```python
from build123d import *

# Parameters (mm, degrees)
SKETCH1_W           = 19.81
SKETCH1_H           = 6.73
BOSS_EXTRUDE1_DEPTH = 7.37
SKETCH2_W           = 1.57
SKETCH2_H           = 0.25
BOSS_EXTRUDE2_DEPTH = 2.79
CHAMFER1_SIZE       = 0.4
SKETCH3_W           = 17.31
SKETCH3_H           = 4.23
CUT_EXTRUDE1_DEPTH  = 6
FILLET1_R           = 0.5


with BuildPart() as part:
    # Sketch1 → Boss-Extrude1 (new body)
    with BuildSketch(Plane(origin=(0, 0, 0), x_dir=(1, 0, 0), z_dir=(0, 1, 0))):
        with Locations((9.905, 3.365)):
            Rectangle(SKETCH1_W, SKETCH1_H)
    extrude(amount=BOSS_EXTRUDE1_DEPTH)

    # Sketch2 → Boss-Extrude2 (add)
    with BuildSketch(Plane.XZ):
        with Locations((3.17, -5.065)):
            Rectangle(SKETCH2_W, SKETCH2_H)
        with Locations((3.17, -1.665)):
            Rectangle(SKETCH2_W, SKETCH2_H)
        with Locations((16.64, -1.665)):
            Rectangle(SKETCH2_W, SKETCH2_H)
        with Locations((16.64, -5.065)):
            Rectangle(SKETCH2_W, SKETCH2_H)
    extrude(amount=BOSS_EXTRUDE2_DEPTH)

    # Chamfer1
    chamfer1_edges = [part.edges().sort_by_distance(p)[0] for p in [
        (3.955, -2.79, -5.065),
        (2.385, -2.79, -5.065),
        (3.955, -2.79, -1.665),
        (2.385, -2.79, -1.665),
        (17.425, -2.79, -1.665),
        (15.855, -2.79, -1.665),
        (17.425, -2.79, -5.065),
        (15.855, -2.79, -5.065),
    ]]
    chamfer(chamfer1_edges, length=CHAMFER1_SIZE)

    # Sketch3 → Cut-Extrude1 (cut)
    with BuildSketch(Plane(origin=(0, 7.37, 0), x_dir=(1, 0, 0), z_dir=(0, 1, 0))):
        with Locations((9.905, 3.365)):
            Rectangle(SKETCH3_W, SKETCH3_H)
    extrude(amount=-CUT_EXTRUDE1_DEPTH, mode=Mode.SUBTRACT)

    # Fillet1
    fillet1_edges = [part.edges().sort_by_distance(p)[0] for p in [
        (19.81, 7.37, -3.365),
        (9.905, 7.37, -6.73),
        (0, 7.37, -3.365),
        (0, 3.685, -6.73),
        (19.81, 3.685, -6.73),
        (19.81, 3.685, 0),
        (0, 3.685, 0),
        (9.905, 7.37, 0),
    ]]
    fillet(fillet1_edges, radius=FILLET1_R)


solid = part.part
```
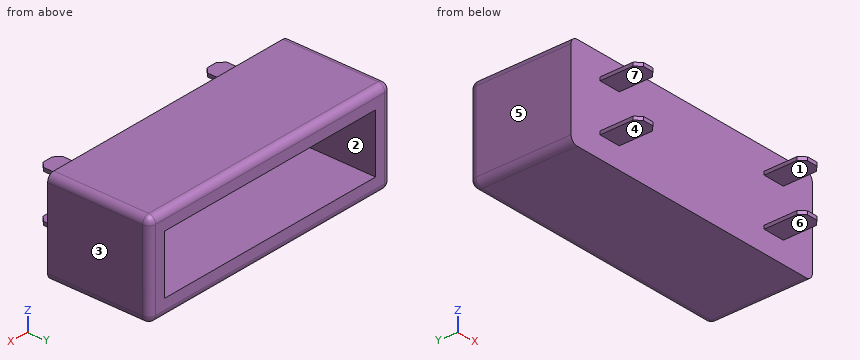
CAD build for the part. Positions are in the model's coordinates, mm. Face numbers are marked on the shaded views. A direction names the side the tool comes from. Round coordinates to 2 decimals unless told otherwise and drop trailing zeros. Order: outer loops, then holes, each group sorted by start corner. A loop starts at its lowest first (then second) coordinate and runs counter-clockwise, first axis right, second up. Notation, with made-up numbers: (-31, -26) - (11, -26) arc R13 cw to (11, -3) - close; hole circle Ø9 at (5, -5.5). An arc over 180 degrees is marked (long way). Answer as CSV lines item,"result". Start each with the question number.
1. Pin check, flat tips, straight feed: pin 1 (0.5 mm diameter, centred on x = 3.5, y = -1.5, fed in from -Z); pin 2 (1.5 mm diameter, centred on y = -1, z = -3, fed in from +X); pin 3 (1.3 mm diameter, centred on x = 16.5, y = -1.5, fed in from +Z). Stop position of each tip, or through.
2. Saw through at A-A, the plane y = 2.75. Write the cut outline in (x, z), and give its area (3 significant figures).
3. Saw through at B-B, the plane x = 6.5. Write the cut outline in (y, z), and give its area (3 significant figures).
4. Tool access for the marked faces 1, 2, 3 and 4: list every direction of +Z, -Z, +X, -X, +Y, -Y with a clear straight run to the whole face (end or side of a thin tool).
5. Drill centre lines: L1, parallel to X at y = 5, z = -4.25; L2, parallel to Z at x = 17, y = 4.75; L3, parallel to Y at x = 9.5, z = -4. Where is each one in solid material? Low to high. Write a range as [from, to].
6. Pull direction Z, two halves, no side cores. Call the marked faces 5, 6 and 7: +Z half, -Z half, draft (parallel to the pull), parting line (faces both ways), or undercut.
7. Saw through at C-C, the plane y = -0.25. Write the cut outline in (x, z) (3 decimals).
8. Saw through at D-D, the plane z = -4.25. Write the cut outline in (x, y).
Model answer:
1,pin 1,"stops at z = -5.19"
1,pin 2,"passes through"
1,pin 3,"stops at z = -1.54"
2,outline,"(0, -6.23) arc R0.5 ccw to (0.5, -6.73) - (19.31, -6.73) arc R0.5 ccw to (19.81, -6.23) - (19.81, -0.5) arc R0.5 ccw to (19.31, 0) - (0.5, 0) arc R0.5 ccw to (0, -0.5) - close; hole (1.25, -5.48) - (18.56, -5.48) - (18.56, -1.25) - (1.25, -1.25) - close"
2,area,"59.9 mm²"
3,outline,"(0, -6.73) - (6.87, -6.73) arc R0.5 ccw to (7.37, -6.23) - (7.37, -5.48) - (1.37, -5.48) - (1.37, -1.25) - (7.37, -1.25) - (7.37, -0.5) arc R0.5 ccw to (6.87, 0) - (0, 0) - close"
3,area,"24.1 mm²"
4,face 1,"+X, -X, -Y"
4,face 2,"+Y"
4,face 3,"+Z, -Z, +X, +Y, -Y"
4,face 4,"-Z, +X, -X, -Y"
5,L1,"x = [0, 1.25], [18.56, 19.81]"
5,L2,"z = [-6.73, -5.48], [-1.25, 0]"
5,L3,"y = [0, 1.37]"
6,face 5,"draft"
6,face 6,"-Z half"
6,face 7,"undercut"
7,outline,"(2.385, -5.19) - (3.955, -5.19) - (3.955, -4.94) - (2.385, -4.94) - close; (2.385, -1.79) - (3.955, -1.79) - (3.955, -1.54) - (2.385, -1.54) - close; (15.855, -5.19) - (17.425, -5.19) - (17.425, -4.94) - (15.855, -4.94) - close; (15.855, -1.79) - (17.425, -1.79) - (17.425, -1.54) - (15.855, -1.54) - close"
8,outline,"(0, 0) - (19.81, 0) - (19.81, 6.87) arc R0.5 ccw to (19.31, 7.37) - (18.56, 7.37) - (18.56, 1.37) - (1.25, 1.37) - (1.25, 7.37) - (0.5, 7.37) arc R0.5 ccw to (0, 6.87) - close"
